Read the model definition and answer for the solid it produces. Units are mm, in the model's axes. Coordinates: 2 decimals unless noted, no trailing zeros.
from build123d import *

# Parameters (mm, degrees)
EXTRUDE_DEPTH = 10


with BuildPart() as part:
    # path4181 → Extrude (new body)
    with BuildSketch(Plane(origin=(19.999989, -22.71163, 0), x_dir=(0, -1, 0), z_dir=(0, 0, -1))):
        with BuildLine():
            add(Edge.make_bspline(
                [(22.570525, -1.969483), (7.304641, -1.805358)],
                knots=[0, 0, 54.094838, 54.094838], degree=1))
            add(Edge.make_bspline(
                [(7.304641, -1.805358), (12.393269, 19.85894)],
                knots=[0, 0, 78.852395, 78.852395], degree=1))
            add(Edge.make_bspline(
                [(12.393269, 19.85894), (0.246224, 0.820617)],
                knots=[0, 0, 80.019804, 80.019804], degree=1))
            add(Edge.make_bspline(
                [(0.246224, 0.820617), (3.693359, 17.561211)],
                knots=[0, 0, 60.561559, 60.561559], degree=1))
            add(Edge.make_bspline(
                [(3.693359, 17.561211), (-8.781986, 3.28247)],
                knots=[0, 0, 67.184379, 67.184379], degree=1))
            add(Edge.make_bspline(
                [(-8.781986, 3.28247), (-6.648045, 15.755852)],
                knots=[0, 0, 44.839145, 44.839145], degree=1))
            add(Edge.make_bspline(
                [(-6.648045, 15.755852), (-22.570525, -0.492372)],
                knots=[0, 0, 80.607717, 80.607717], degree=1))
            add(Edge.make_bspline(
                [(-22.570525, -0.492372), (-7.632941, -12.80163)],
                knots=[0, 0, 68.58375, 68.58375], degree=1))
            add(Edge.make_bspline(
                [(-7.632941, -12.80163), (-10.09518, -3.446593)],
                knots=[0, 0, 34.276682, 34.276682], degree=1))
            add(Edge.make_bspline(
                [(-10.09518, -3.446593), (1.066971, -15.919976)],
                knots=[0, 0, 59.309806, 59.309806], degree=1))
            add(Edge.make_bspline(
                [(1.066971, -15.919976), (-0.902821, -6.072568)],
                knots=[0, 0, 35.583612, 35.583612], degree=1))
            add(Edge.make_bspline(
                [(-0.902821, -6.072568), (9.766881, -19.85894)],
                knots=[0, 0, 61.770178, 61.770178], degree=1))
            add(Edge.make_bspline(
                [(9.766881, -19.85894), (7.304641, -5.744322)],
                knots=[0, 0, 50.7677, 50.7677], degree=1))
            add(Edge.make_bspline(
                [(7.304641, -5.744322), (22.570525, -6.072568)],
                knots=[0, 0, 54.104215, 54.104215], degree=1))
            add(Edge.make_bspline(
                [(22.570525, -6.072568), (22.570525, -1.969483)],
                knots=[0, 0, 14.538494, 14.538494], degree=1))
        make_face()
    extrude(amount=EXTRUDE_DEPTH)


solid = part.part
Q1. Each of these flat-tipped pins is pushed along its axis until it touches: P1, Ø2, axis at y = -9, z = -8.5, coming from the -X side; P2, Ø1, axis at y = -39.5, z = -1.5, coming from the +X side; P3, Ø4, axis at x = 30.5, z = -3.5, coming from the -Y side. Where does it stop, or does it pass through?
Q2. Straight lines are drawn through the part: L1, parallel to Y at x = 7.5, z = -2.5; L2, parallel to Y at x = 4.5, z = -4.75; L3, parallel to Y at x = 4, z = -9.25. For each, find the intervals that lie inside material, in ascending order.
Q3. The part is cut by section A-A, the plane x = 7.5. State how many separate pieces and enclosed holes the cut face has, then the cut area to 3 significant figures.
Computed values:
1. P1: stops at x = 10.43
1. P2: stops at x = 25.96
1. P3: stops at y = -31.19
2. L1: y = -33.38 to -30.41, -25.36 to -21.98, -15.51 to -12.87
2. L2: y = -34.08 to -32.32, -25.98 to -24.6, -16.02 to -15.81
2. L3: y = -34.2 to -32.64, -26.08 to -25.04
3. separate pieces: 3
3. enclosed holes: 0
3. area: 89.8 mm2
